Check sheet for the modelled part. Datum: model origin and axes. Units: mm. A direction names the side the tool comes from. Round coordinates to 2 decimals unless told otherwise and drop trailing zeros. Loops run counter-clockwise (first coordinate to the right, second up) from the corner with the lowest first, then second, coordinate; pieces in that order, holes last. Notation, with made-up numbers: (71.25, 79.5) - (96.25, 79.5) arc R17 cw to (96.25, 110.5) - close; hole circle Ø7 at (31.5, 62.25). An arc over 180 degrees is marked (long way). Answer in a Markdown table with one row per item. Add a question column.
(1) Thickness scan on line 1 along X through (y, z) = (-54, 3); line 2 along X through (y, z) = (-24, 0.5); line 3 along Z through (x, y) = (-38.5, -46). Record the ranges inside material, lowest first.
(2) Gauge pin test, flat ends, axial feed: pin 1 (0.5 mm diameter, centred on y = -39.5, z = 6.5, fed in from +X); pin 2 (15.5 mm diameter, centred on x = -24.5, y = -25, fed in from -Z); pin 3 (1.1 mm diameter, centred on x = -8, z = 6.5, fed in from -Y). Record the tip position at first contact, or that the pin passes through.
(3) Access from +Z, -Z, +X, -X, +Y, -Y to the whole of each face (thin tool, end or side, straight path). Record for faces 4 (the flat face through (-55, -30, 5)), 5 (the flat face through (-37, -21, 7)).
(4) Cross-section at C-C on z = 2.5. Enter the section's corners in (x, y), then the cut area to 3 significant figures.
(5) Cross-section at A-A on x = -39. Enter the section's corners in (y, z).
(6) Cross-section at B-B on y = -40.5. Enter the section's corners in (x, z).
(7) Mould release check, pull along Z, two halves, no side actions. Record for faces 1 (the flat face through (-38, -7, 1)), 2 (the flat face through (-52, -20, 0)), 3 (the flat face through (0, -6.6, 6.1)): +Z half, -Z half, draft (parallel to the pull), parting line (faces both ways), or undercut.
from build123d import *

# Parameters (mm, degrees)
F3_R = 5
F4_R = 5


with BuildPart() as f2:
    # F2: sweep along a path in F1
    with BuildLine(Plane.XY) as f2_path:
        Line((0, 1.6581159234), (-60, 1.6581159234))
        Line((-60, 1.6581159234), (-60, -58.3418840766))
    # F0 (on Right) → F2 (sweep)
    with BuildSketch(Plane.YZ):
        Polygon((1.6581159234, 7), (-24.3418840766, 7), (-24.3418840766, 6), (-7.3418840766, 6), (0.6581159234, 4), (0.6581159234, 1), (-8.3418840766, 1), (-8.3418840766, 0), (1.6581159234, 0), align=None)
    sweep(path=f2_path.line, transition=Transition.RIGHT)

    # F3
    f3_edges = [f2.edges().sort_by_distance(p)[0] for p in [
        (-59, 0.658116, 2.5),
    ]]
    fillet(f3_edges, radius=F3_R)

    # F4
    f4_edges = [f2.edges().sort_by_distance(p)[0] for p in [
        (-34, -24.341884, 6.5),
        (-60, 1.658116, 3.5),
    ]]
    fillet(f4_edges, radius=F4_R)


solid = f2.part
Answers:
| question | item | result |
|---|---|---|
| 1 | line 1 | x = -60 to -59 |
| 1 | line 2 | x = -60 to -50 |
| 1 | line 3 | z = 6 to 7 |
| 2 | pin 1 | stops at x = -34 |
| 2 | pin 2 | stops at z = 6 |
| 2 | pin 3 | stops at y = -24.34 |
| 3 | face 4 | +X, -Y |
| 3 | face 5 | +Z, +X, -X, +Y, -Y |
| 4 | outline | (-60, -58.34) - (-59, -58.34) - (-59, -4.34) arc R5 cw to (-54, 0.66) - (0, 0.66) - (0, 1.66) - (-55, 1.66) arc R5 ccw to (-60, -3.34) - close |
| 4 | area | 119 mm^2 |
| 5 | outline | (-58.34, 6) - (-7.34, 6) - (0.66, 4) - (0.66, 1) - (-8.34, 1) - (-8.34, 0) - (1.66, 0) - (1.66, 7) - (-58.34, 7) - close |
| 6 | outline | (-60, 0) - (-50, 0) - (-50, 1) - (-59, 1) - (-59, 4) - (-51, 6) - (-34, 6) - (-34, 7) - (-60, 7) - close |
| 7 | face 1 | undercut |
| 7 | face 2 | -Z half |
| 7 | face 3 | draft |
